Could you check a few things on this model? Use its own coordinates, in mm. Face numbers are marked on the shaded views. A direction names the side the tool comes from. Give positions to 0.01 mm unless a question says otherwise; leave off trailing zeros. Order: outer loops, then holes, each group sorted by start corner. A loop starts at its lowest first (then second) coordinate and runs counter-clockwise, first axis right, second up. Notation, with made-up numbers: (28.5, 72.5) -> (72.5, 72.5) arc R34 ccw to (72.5, 104.5) -> close; hole circle Ø8 at (39.5, 76.5). An arc over 180 degrees is marked (long way). Use one line per item in the form item = value. Start each with the question number.
Autodesk Inventor part; units mm, degrees
ref_plane "YZ Plane" through (0, 0, 0) normal (1, 0, 0) x (0, 1, 0)
ref_plane "XZ Plane" through (0, 0, 0) normal (0, 1, 0) x (-1, 0, 0)
ref_plane "XY Plane" through (0, 0, 0) normal (0, 0, 1) x (1, 0, 0)
sketch "Sketch1" plane through (0, 0, 0) normal (0, 0, 1) x (1, 0, 0)
  line L0 (31.75, -44.45) -> (-31.75, -44.45)
  line L1 (-31.75, -44.45) -> (-31.75, 44.45)
  line L2 (-31.75, 44.45) -> (31.75, 44.45)
  line L3 (31.75, 44.45) -> (31.75, -44.45)
  line L4 (31.75, -44.45) -> (-31.75, 44.45) construction
  line L5 (-31.75, -44.45) -> (31.75, 44.45) construction
  line L6 (-31.75, 0) -> (31.75, 0)
  line L7 (-31.75, 44.45) -> (31.75, 0)
  line L8 (-31.75, 0) -> (31.75, 44.45)
  circle A0 centre (0, 22.225) radius 11.43
  point P0 (0, 0)
  dimension "d0" = 63.5
  dimension "d1" = 44.45
  dimension "d2" = 22.86
extrude "Extrusion1" add sketch "Sketch1" along normal blind 3.175 contours L0 L1 L6 L3 | A0 L8 L7 | L7 L8 A0 | A0 L7 L8 | L8 L7 A0
sketch "Sketch2" plane through (0, 0, 3.175) normal (0, 0, 1) x (1, 0, 0)
  line L0 (31.75, -44.45) -> (31.75, 0)
  line L1 (31.75, 0) -> (-31.75, 0)
  line L2 (-31.75, 0) -> (-31.75, -44.45)
  line L3 (-31.75, -44.45) -> (31.75, -44.45)
  line L4 (-31.75, 44.45) -> (31.75, 44.45)
  line L5 (31.75, 44.45) -> (31.75, -44.45)
  line L6 (31.75, -44.45) -> (-31.75, -44.45)
  line L7 (-31.75, -44.45) -> (-31.75, 44.45)
  line L8 (-31.75, 44.45) -> (31.75, -44.45) construction
  line L9 (31.75, 44.45) -> (-31.75, -44.45) construction
  point P0 (0, 0)
extrude "Extrusion2" add sketch "Sketch2" along normal blind 3.175
sketch "Sketch3" plane through (0, 0, 6.35) normal (0, 0, 1) x (1, 0, 0)
  circle A0 centre (0, -0.4493) radius 54.991
  line L0 (0, -0.4493) -> (0, 0)
  line L1 (31.75, -44.45) -> (31.75, 44.45)
  line L2 (31.75, 44.45) -> (-31.75, 44.45)
  line L3 (-31.75, 44.45) -> (-31.75, -44.45)
  line L4 (-31.75, -44.45) -> (31.75, -44.45)
  line L5 (-31.75, -44.45) -> (31.75, -44.45)
  line L6 (0, 44.45) -> (0, -44.45)
  line L7 (31.75, 0) -> (-31.75, 0)
  line L8 (-31.75, 0) -> (31.75, 0)
  line L9 (12.7, 12.7) -> (-12.7, 12.7)
  line L10 (-12.7, 12.7) -> (-12.7, 44.45)
  line L11 (-12.7, 44.45) -> (12.7, 44.45)
  line L12 (12.7, 44.45) -> (12.7, 12.7)
  line L13 (12.7, 12.7) -> (-12.7, 44.45) construction
  line L14 (-12.7, 12.7) -> (12.7, 44.45) construction
  line L15 (-33.655, 6.35) -> (-8.255, 6.35)
  line L16 (-8.255, 6.35) -> (-8.255, -16.51)
  line L17 (-8.255, -16.51) -> (-33.655, -16.51)
  line L18 (-33.655, -16.51) -> (-33.655, 6.35)
  line L19 (-8.255, 6.35) -> (31.75, 6.35)
  line L20 (-8.255, -12.7) -> (-3.175, -12.7)
  line L21 (-3.175, -12.7) -> (-3.175, -44.45)
  line L22 (-20.955, 6.35) -> (-20.955, 12.7)
  line L23 (-20.955, 12.7) -> (-31.75, 12.7)
  line L24 (3.175, 6.35) -> (3.175, -44.45)
  point P0 (0, -55.4403)
  point P1 (0, 28.575)
  point P2 (3.175, -44.45)
  point P3 (-3.175, -44.45)
  point P4 (-31.75, -16.51)
  dimension "d8" = 109.982
  dimension "d9" = 25.4
  dimension "d10" = 31.75
  dimension "d11" = 25.4
  dimension "d12" = 8.255
  dimension "d13" = 6.35
  dimension "d14" = 22.86
  dimension "d15" = 5.08
  dimension "d16" = 19.05
  dimension "d17" = 6.35
extrude "Extrusion3" add sketch "Sketch3" along normal blind 12.7 contours L1 L19 L6 L9 L12 L2 | L2 L10 L9 L6 L19 L15 L22 L23 L3 | L1 L7 L24 L19 | L1 L4 L24 L7 | L17 L16 L20 L21 L4 L3
sketch "Sketch4" plane through (0, 0, 19.05) normal (0, 0, 1) x (1, 0, 0)
  line L0 (-20.955, 12.7) -> (-20.955, 6.35)
  line L1 (-20.955, 6.35) -> (3.175, 6.35)
  line L2 (3.175, 6.35) -> (3.175, -44.45)
  line L3 (3.175, -44.45) -> (31.75, -44.45)
  line L4 (31.75, -44.45) -> (31.75, 44.45)
  line L5 (31.75, 44.45) -> (12.7, 44.45)
  line L6 (12.7, 44.45) -> (12.7, 12.7)
  line L7 (12.7, 12.7) -> (-12.7, 12.7)
  line L8 (-12.7, 12.7) -> (-12.7, 44.45)
  line L9 (-12.7, 44.45) -> (-31.75, 44.45)
  line L10 (-31.75, 44.45) -> (-31.75, 12.7)
  line L11 (-31.75, 12.7) -> (-20.955, 12.7)
  line L12 (-3.175, -12.7) -> (-8.255, -12.7)
  line L13 (-8.255, -12.7) -> (-8.255, -16.51)
  line L14 (-8.255, -16.51) -> (-31.75, -16.51)
  line L15 (-31.75, -16.51) -> (-31.75, -44.45)
  line L16 (-31.75, -44.45) -> (-3.175, -44.45)
  line L17 (-3.175, -44.45) -> (-3.175, -12.7)
  line L18 (3.175, -44.45) -> (3.175, 6.35)
  line L19 (3.175, 6.35) -> (-20.955, 6.35)
  line L20 (-20.955, 6.35) -> (-20.955, 12.7)
  line L21 (-20.955, 12.7) -> (-31.75, 12.7)
  line L22 (-31.75, 12.7) -> (-31.75, -16.51)
  line L23 (-31.75, -16.51) -> (-8.255, -16.51)
  line L24 (-8.255, -16.51) -> (-8.255, -12.7)
  line L25 (-8.255, -12.7) -> (-3.175, -12.7)
  line L26 (-3.175, -12.7) -> (-3.175, -44.45)
  line L27 (-3.175, -44.45) -> (3.175, -44.45)
  line L28 (31.75, 0) -> (-31.75, 0)
  line L29 (-31.75, -25.4) -> (31.75, -25.4)
  line L30 (0, 0) -> (0, -44.45)
  line L31 (12.7, -26.9875) -> (-12.7, -26.9875)
  line L32 (-12.7, -26.9875) -> (-12.7, -23.8125)
  line L33 (-12.7, -23.8125) -> (12.7, -23.8125)
  line L34 (12.7, -23.8125) -> (12.7, -26.9875)
  line L35 (12.7, -26.9875) -> (-12.7, -23.8125) construction
  line L36 (-12.7, -26.9875) -> (12.7, -23.8125) construction
  point P0 (0, -25.4)
  dimension "d20" = 25.4
  dimension "d21" = 3.175
  dimension "d22" = 25.4
extrude "Extrusion4" cut sketch "Sketch4" against normal blind 9.525 contours L33 L34 L29 L2 | L2 L29 L30 L33 | L30 L29 L17 L33 | L29 L34 L31 L2 | L2 L31 L30 L29 | L32 L33 L17 L29 | L29 L17 L31 L32 | L30 L31 L17 L29
sketch "Sketch5" plane through (0, 0, 0) normal (0, 1, 0) x (-1, 0, 0)
  line L0 (-31.75, 3.175) -> (31.75, 3.175)
  line L1 (31.75, 3.175) -> (31.75, 19.05)
  line L2 (12.7, 19.05) -> (31.75, 19.05)
  line L3 (12.7, 6.35) -> (12.7, 19.05)
  line L4 (-12.7, 6.35) -> (12.7, 6.35)
  line L5 (-12.7, 6.35) -> (-12.7, 19.05)
  line L6 (-31.75, 19.05) -> (-12.7, 19.05)
  line L7 (-31.75, 3.175) -> (-31.75, 19.05)
  circle A0 centre (0, -25.4) radius 63.5
  line L8 (0, 0) -> (0, -25.4)
  circle A1 centre (0, -25.4) radius 114.3
  line L9 (0, -25.4) -> (114.3, -25.4)
  line L10 (0, -25.4) -> (0, 88.9)
  point P0 (0, 38.1)
  point P1 (63.5, -25.4)
  dimension "d25" = 28.575
  dimension "d26" = 127
  dimension "d27" = 50.8
revolve "Revolution1" cut sketch "Sketch5" angle 360 about axis through (0, 0, -25.4) along (0, 0, 1) picked at (44.2136, 61.1262) contours L10 A1 L9 A0
sketch "Sketch7" plane through (3.175, -44.45, 6.35) normal (-1, 0, 0) x (0, 0, 1)
  arc A0 (0.6288, 0) -> (12.7, 12.0712) centre (-31.75, 44.45) ccw
  line L0 (-6.35, 0) -> (0.6288, 0)
  line L1 (-6.35, 0) -> (-6.35, 44.45)
  line L2 (-6.35, 44.45) -> (-3.175, 44.45)
  line L3 (-3.175, 44.45) -> (-3.175, 88.9)
  line L4 (-3.175, 88.9) -> (0.6288, 88.9)
  arc A1 (12.7, 76.8288) -> (0.6288, 88.9) centre (-31.75, 44.45) ccw
  line L5 (12.7, 12.0712) -> (12.7, 76.8288)
  line L6 (0, 50.8) -> (12.7, 50.8)
  line L7 (12.7, 20.6375) -> (3.175, 20.6375)
  line L8 (12.7, 17.4625) -> (3.175, 17.4625)
  circle A2 centre (6.35, 44.45) radius 6.35
  circle A3 centre (4.7625, 19.05) radius 1.5875
  line L9 (3.175, 20.6375) -> (3.175, 17.4625)
  line L10 (12.7, 20.6375) -> (3.175, 20.6375)
  circle A4 centre (6.35, 44.45) radius 2.4478
  dimension "d37" = 12.7
  dimension "d38" = 3.175
extrude "Extrusion5" cut sketch "Sketch7" along normal mid plane 38.1 contours A3 | A2 | A4
properties part number "bunny head anchor"
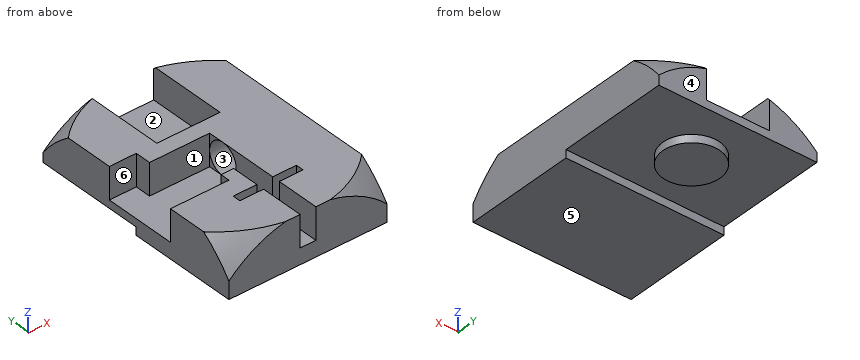
(1) Please list where these lines run through material, in increasing order: probe 1 along Y at (x, z) = (9.75, 12.7); probe 2 along Z at (x, y) = (16.5, -25.4) (3 decimals); probe 3 along Y at (x, z) = (-6.5, 9).
(2) Imagine slicing it at B-B (z = 8.5). Write out the boundary of the cut face in (x, y) (3 decimals), plus the area to 3 significant figures.
(3) We'd pull the mould along Y, two halves only. Please class the marked faces 4, 5 and 6: pulls with the +Y half, pulls with the -Y half, needs draft (parallel to the pull), parting line crosses it, or undercut.
(4) I'm going to push flat-ended pins straight in: pin 1 Ø12 at (x, y) = (-18, 6.5) entering from -Z (3 decimals); pin 2 Ø3 at (x, z) = (-8, 12.5) entering from +Y; pin 3 Ø10.5 at (x, y) = (-20.5, -11) entering from +Z. Where does each tip first touch, or does it pass through?
(5) Imagine slicing it at C-C (x = 0). Write out the boundary of the cut face in (y, z) (3 decimals).
(6) Imagine slicing it at A-A (y = -20). Write out the boundary of the cut face in (x, z) (3 decimals).
(7) Which directions (+Z, -Z, +X, -X, +Y, -Y) give clear straight access to the entire face, cutting with the end or side of a thin tool? Please do the marked faces 1, 2 and 3.
Calculated:
q1.probe_1 = -44.45 to -26.99, -23.81 to -6.35, 6.35 to 12.7
q1.probe_2 = 0 to 9.525, 12.7 to 19.05
q1.probe_3 = -44.45 to -12.7, 6.35 to 12.7
q2.outline = (-31.75, -43.301) arc R53.694 ccw to (-30.12, -44.45) -> (-3.175, -44.45) -> (-3.175, -12.7) -> (-8.255, -12.7) -> (-8.255, -16.51) -> (-31.75, -16.51) -> close; (-31.75, 12.7) -> (-20.955, 12.7) -> (-20.955, 6.35) -> (3.175, 6.35) -> (3.175, 4.763) -> (22.225, 4.763) -> (22.225, -4.763) -> (3.175, -4.763) -> (3.175, -44.45) -> (30.12, -44.45) arc R53.694 ccw to (31.75, -43.301) -> (31.75, 43.301) arc R53.694 ccw to (30.12, 44.45) -> (12.7, 44.45) -> (12.7, 12.7) -> (-12.7, 12.7) -> (-12.7, 44.45) -> (-30.12, 44.45) arc R53.694 ccw to (-31.75, 43.301) -> close
q2.area = 3,630 mm2
q3.face_4 = pulls with the +Y half
q3.face_5 = needs draft
q3.face_6 = undercut
q4.pin_1 = 3.175
q4.pin_2 = 12.7
q4.pin_3 = 6.35
q5.outline = (-44.45, 0) -> (0, 0) -> (0, 3.175) -> (10.795, 3.175) -> (10.795, 0) -> (33.655, 0) -> (33.655, 3.175) -> (44.45, 3.175) -> (44.45, 6.35) -> (12.7, 6.35) -> (12.7, 19.05) -> (6.35, 19.05) -> (6.35, 6.35) -> (-44.45, 6.35) -> close
q6.outline = (-31.75, 0) -> (31.75, 0) -> (31.75, 19.05) -> (3.175, 19.05) -> (3.175, 6.35) -> (-3.175, 6.35) -> (-3.175, 19.05) -> (-31.75, 19.05) -> close
q7.face_1 = +Z, -X
q7.face_2 = +Z, +Y
q7.face_3 = -X
